Work out the finished part from the listing and answer in its coordinate system (mm). Give positions to 0.01 mm unless a question says otherwise; leave off trailing zeros. Loops run counter-clockwise (first coordinate to the right, second up) from the corner with the lowest first, then second, coordinate; pieces in that order, holes last. Notation, with made-up numbers: (26, 14) - (71, 14) arc R23 cw to (71, 33) - close; hole circle Ø2 at (40, 13). An arc over 180 degrees is marked (long way). One line per question, with ' | ' between items.
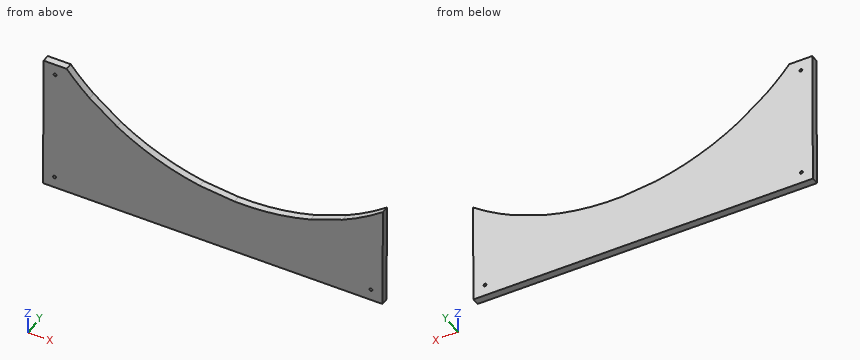
from build123d import *

# Parameters (mm, degrees)
SKETCH1_R           = 1.25
BOSS_EXTRUDE1_DEPTH = 6.35


with BuildPart() as part:
    # Sketch1 → Boss-Extrude1 (new body)
    with BuildSketch(Plane(origin=(0, 0, 0), x_dir=(1, 0, 0), z_dir=(0, 1, 0))):
        with BuildLine():
            Line((19.999792019, 0.091209594), (0, 0))
            Line((0, 0), (-0.547257564, 119.998752115))
            Line((-0.547257564, 119.998752115), (294.449674718, 121.344093627))
            Line((294.449674718, 121.344093627), (294.86012216, 31.344093627))
            ThreePointArc((294.86012216, 31.344093627), (277.870515385, 42.942471612), (259.779400189, 52.734338707))
            Line((259.779400189, 52.734338707), (231.756657954, 63.5857763))
            ThreePointArc((231.756657954, 63.5857763), (199.118358441, 70.566953886), (165.773569429, 72.023141123))
            Line((165.773569429, 72.023141123), (135.773569429, 68.543550593))
            ThreePointArc((135.773569429, 68.543550593), (98.326093616, 57.414966094), (63.756361786, 39.21901932))
            Line((63.756361786, 39.21901932), (40.005697256, 20.884351348))
            ThreePointArc((40.005697256, 20.884351348), (29.627268731, 10.849040712), (19.999792019, 0.091209594))
        make_face()
        with Locations(Location((9.498243242, 110.044460902, 0), (0, 0, 270))):
            Circle(SKETCH1_R, mode=Mode.SUBTRACT)
        with Locations(Location((9.954291213, 10.045500807, 0), (0, 0, 270))):
            Circle(SKETCH1_R, mode=Mode.SUBTRACT)
        with Locations(Location((284.495383506, 111.298592821, 0), (0, 0, 270))):
            Circle(SKETCH1_R, mode=Mode.SUBTRACT)
    extrude(amount=BOSS_EXTRUDE1_DEPTH)


solid = part.part
1. Consider L1, parallel to X at y = 3.5, z = -35; L2, parallel to X at y = 4.75, z = -46.5; L3, parallel to Z at x = 165.5, y = 3.75. Determine where each line is inside the solid, lowest interval first.
Evaluation:
L1: -0.16 to 58.29, 289.9 to 294.84 | L2: -0.21 to 75.7, 271.8 to 294.79 | L3: -120.76 to -71.99
2. Find section C-C on z = -15. Write down the section's boundary in (x, y).
Evaluation:
outline: (-0.07, 0) - (33.74, 0) - (33.74, 6.35) - (-0.07, 6.35) - close
3. Find section B-B on x = 130. Write down the section's boundary in (y, z).
Evaluation:
outline: (0, -120.59) - (6.35, -120.59) - (6.35, -67.34) - (0, -67.34) - close
4. Flat-ended cylindrical pins translate along their axes: pin 1 (2 mm diameter, centred on x = 9.95, z = -10.05, fed in from -Y); pin 2 (3 mm diameter, centred on x = 9.5, z = -110.04, fed in from +Y). Find the tip coordinate at first contact, or state that the pin passes through.
Evaluation:
pin 1: through | pin 2: y = 6.35
5. Find section A-A on y = 1.5. Write down the section's boundary in (x, z), then the cut area to 3 significant figures.
Evaluation:
outline: (-0.55, -120) - (294.45, -121.34) - (294.86, -31.34) arc R200 cw to (259.78, -52.73) - (231.76, -63.59) arc R200 cw to (165.77, -72.02) - (135.77, -68.54) arc R200 cw to (63.76, -39.22) - (40.01, -20.88) arc R200 cw to (20, -0.09) - (0, 0) - close; hole circle Ø2.5 at (9.5, -110.04); hole circle Ø2.5 at (9.95, -10.05); hole circle Ø2.5 at (284.5, -111.3) | area: 20,700 mm2
